Can you work these out from the model? Positions are in its coordinate system, mm. Face numbers are marked on the shaded views. A direction names the side the tool comes from. Round coordinates to 2 decimals unless told otherwise and drop trailing zeros. Order: outer loops, then holes, each group sorted by start corner. A loop starts at its lowest first (then second) coordinate and runs counter-clockwise, first axis right, second up. Notation, with made-up numbers: (38.5, -6) -> (69.5, -6) arc R17 cw to (69.5, 4) -> close; hole circle Ø8 at (85, 43). An arc over 180 degrees is marked (long way). Use a Markdown table: item, result. Add a question column.
Q1. I'm going to push flat-ended pins straight in: pin 1 Ø10 at (y, z) = (-5.5, 41.5) entering from +X; pin 2 Ø6 at (y, z) = (-28, 31.5) entering from +X; pin 3 Ø2 at (x, z) = (-14, 35.5) entering from -Y. Where does each tip first touch, or does it pass through?
Q2. If we section it at A-A on x = -23: List the corners of the cut face in (y, z) for me, plus the area to 3 significant figures.
Q3. For the marked faces 1, 2, 3 and 4, which set-ups out of +Z, -Z, +X, -X, +Y, -Y let a thin tool reach every point of the face, with its end or its side?
Q4. If we section it at B-B on y = -35.5: List the corners of the cut face in (x, z) for me.
Q5. If we section it at C-C on y = -3.5: List the corners of the cut face in (x, z) for me, plus the area to 3 significant figures.
Q6. We'd pull the mould along Y, two halves only. Please class the marked faces 5, 6, 7 and 8: +Y half, -Y half, draft (parallel to the pull), parting line (faces both ways), or undercut.
Q7. I need wall thicknesses on line 1 along X through (y, z) = (-8, 20.5); line 2 along X through (y, z) = (-7, 10.5); line 3 along Y through (x, z) = (-28, 5). Which ranges of each line are inside material? Lowest first, please. Write a range as [from, to].
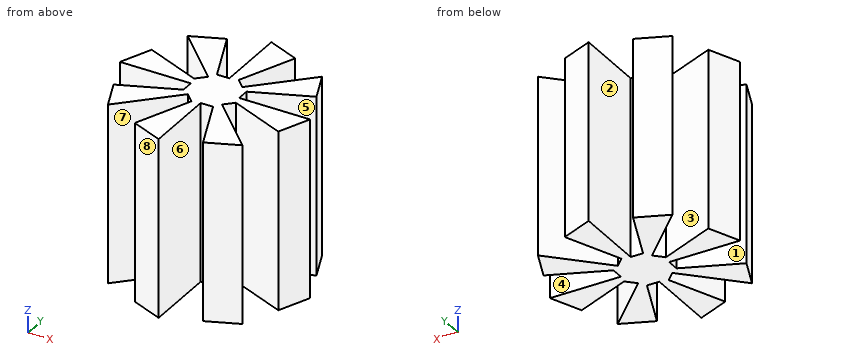
Autodesk Inventor part; units mm, degrees
ref_plane "YZ Plane" through (0, 0, 0) normal (1, 0, 0) x (0, 1, 0)
ref_plane "XZ Plane" through (0, 0, 0) normal (0, 1, 0) x (-1, 0, 0)
ref_plane "XY Plane" through (0, 0, 0) normal (0, 0, 1) x (1, 0, 0)
ref_plane "Płaszczyzna konstrukcyjna1" through (0, 0, 0) normal (0, 0, 1) x (1, 0, 0)
sketch "Szkic1" plane through (0, 0, 0) normal (0, 0, 1) x (1, 0, 0)
  line L0 (8.0251, 3.4329) -> (-11.0866, 11.3492)
  line L1 (-11.0866, 11.3492) -> (-30.1982, 3.4329)
  line L2 (-30.1982, 3.4329) -> (-38.1145, -15.6788)
  line L3 (-38.1145, -15.6788) -> (-30.1982, -34.7904)
  line L4 (-30.1982, -34.7904) -> (-11.0866, -42.7067)
  line L5 (-11.0866, -42.7067) -> (8.0251, -34.7904)
  line L6 (8.0251, -34.7904) -> (15.9414, -15.6788)
  line L7 (15.9414, -15.6788) -> (8.0251, 3.4329)
  point P0 (0, 0)
extrude "Wyciągnięcie proste1" add sketch "Szkic1" along normal blind 50
sketch "Szkic2" plane through (0, 0, 50) normal (0, 0, 1) x (1, 0, 0)
  line L0 (-35.3977, -2.8484) -> (-36.8759, -2.2361)
  line L1 (-31.4727, 0.356) -> (-35.1682, 1.8867)
  line L2 (8.0251, 3.4329) -> (-11.0866, 11.3492) construction
  line L3 (8.0251, 3.4329) -> (-30.1982, -34.7904) construction
  line L4 (-11.0866, 11.3492) -> (-30.1982, 3.4329) construction
  line L5 (-11.0866, -42.7067) -> (8.0251, -34.7904) construction
  line L6 (-30.1982, 3.4329) -> (8.0251, -34.7904) construction
  line L7 (-30.1982, 3.4329) -> (-38.1145, -15.6788)
  line L8 (-30.1982, 3.4329) -> (-15.8633, -10.902)
  line L9 (-15.8633, -10.902) -> (-18.3147, -13.3534)
  line L10 (-18.3147, -13.3534) -> (-34.3927, -6.6936)
  line L11 (-30.1982, 3.4329) -> (-34.3927, -6.6936)
  line L12 (-38.1145, -15.6788) -> (-30.1982, -34.7904)
  line L13 (-34.0232, -6.8467) -> (-37.6815, -15.6788)
  line L14 (-38.1145, -15.6788) -> (-11.0866, -15.6788)
  point P0 (0, 0)
  dimension "d7" = 0.4
extrude "Wyciągnięcie proste2" cut sketch "Szkic2" against normal through all
sketch "Szkic3" plane through (0, 0, 50) normal (0, 0, 1) x (1, 0, 0)
  line L0 (8.0251, 3.4329) -> (-11.0866, 11.3492) construction
  line L1 (-30.1982, -34.7904) -> (-11.0866, -42.7067) construction
  line L2 (8.0251, 3.4329) -> (-30.1982, -34.7904) construction
  line L3 (8.0251, -34.7904) -> (-30.1982, 3.4329) construction
  point P0 (0, 0)
  point P1 (-11.0866, -15.6788)
pattern_circular "Szyk kołowy1" count 8 over 360 about axis through (-11.0866, -15.6788, 50) along (0, 0, 1) of "Wyciągnięcie proste2"
properties part number "dopychacz"
Answer below:
| question | item | result |
|---|---|---|
| 1 | pin 1 | x = 11.38 |
| 1 | pin 2 | x = 4.23 |
| 1 | pin 3 | y = -41.48 |
| 2 | outline | (-27.59, 0) -> (-21.28, 0) -> (-21.28, 50) -> (-27.59, 50) -> close; (-15.68, 0) -> (-11.41, 0) -> (-11.41, 50) -> (-15.68, 50) -> close; (-3.77, 0) -> (5.98, 0) -> (5.98, 50) -> (-3.77, 50) -> close |
| 2 | area | 1,020 mm² |
| 3 | face 1 | +Z, -Z, -X |
| 3 | face 2 | +Z, -Z, +Y |
| 3 | face 3 | +Z, -Z |
| 3 | face 4 | +Z, -Z, +X |
| 4 | outline | (-18.63, 0) -> (-11.09, 0) -> (-11.09, 50) -> (-18.63, 50) -> close; (-2.21, 0) -> (5.27, 0) -> (5.27, 50) -> (-2.21, 50) -> close |
| 5 | outline | (-23.27, 0) -> (-16.8, 0) -> (-16.8, 50) -> (-23.27, 50) -> close; (-11.09, 0) -> (-6.71, 0) -> (-6.71, 50) -> (-11.09, 50) -> close; (1.09, 0) -> (10.46, 0) -> (10.46, 50) -> (1.09, 50) -> close |
| 5 | area | 1,010 mm² |
| 6 | face 5 | undercut |
| 6 | face 6 | draft |
| 6 | face 7 | undercut |
| 6 | face 8 | -Y half |
| 7 | line 1 | [-34.5, -31.24], [-18.77, -14.94], [-11.09, -8.57], [-3.41, 5.84] |
| 7 | line 2 | [-34.09, -33.65], [-19.77, -15.35], [-11.09, -8.16], [-2.41, 8.25] |
| 7 | line 3 | [-32.59, -23.35], [-15.68, -9.34], [1.23, 3.91] |
